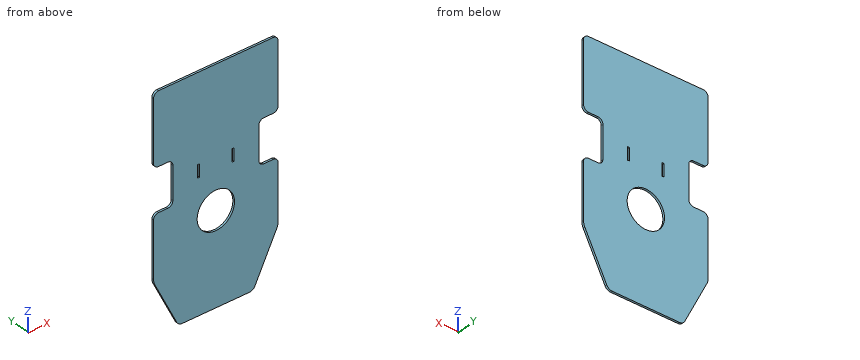
from build123d import *

# Parameters (mm, degrees)
RESSALTO_EXTRUS_O1_DEPTH = 0.8
FILETE6_R                = 2
CHANFRO3_SIZE            = 10
CHANFRO3_SIZE2           = 20
CHANFRO4_SIZE            = 20
CHANFRO4_SIZE2           = 10
FILETE7_R                = 2.5
ESBO_O7_R                = 7.5
CORTE_EXTRUS_O1_DEPTH    = 0.8
CAVIDADE1_START          = -7.3
CAVIDADE1_OUTLINE_W      = 0.8
CAVIDADE1_OUTLINE_H      = 5
CAVIDADE1_DEPTH          = 0.8
CAVIDADE1_START_2        = 6.5
CAVIDADE1_2_OUTLINE_W    = 0.8
CAVIDADE1_2_OUTLINE_H    = 5
CAVIDADE1_2_DEPTH        = 0.8
FILETE8_R                = 5


# Read off the part's stored shape, not the designer's step: Cavidade1
with BuildPart() as part:
    # Esboço1 → Ressalto-extrusão1 (new body)
    with BuildSketch(Plane(origin=(0, 0, 0), x_dir=(1, 0, 0), z_dir=(0, 1, 0))):
        Polygon((-17.25, 45), (-25, 45), (-25, 90), (0, 90), (0, 0), (-25, 0), (-25, 28), (-17.25, 28), align=None)
    ressalto_extrus_o1 = extrude(amount=RESSALTO_EXTRUS_O1_DEPTH)

    # Espelhar8: Ressalto-extrusão1 across plane
    add(ressalto_extrus_o1.mirror(Plane(origin=(0, 0, 0), x_dir=(0, 0, 1), z_dir=(1, 0, 0))))

    # Filete6
    filete6_edges = [part.edges().sort_by_distance(p)[0] for p in [
        (-25, 0.4, -45),
        (-17.25, 0.4, -45),
        (-17.25, 0.4, -28),
        (-25, 0.4, -28),
        (-25, 0.4, 0),
        (25, 0.4, 0),
        (25, 0.4, -28),
        (17.25, 0.4, -28),
        (17.25, 0.4, -45),
        (25, 0.4, -45),
    ]]
    fillet(filete6_edges, radius=FILETE6_R)

    # Chanfro3
    chanfro3_edges = [part.edges().sort_by_distance(p)[0] for p in [
        (-25, 0.4, -90),
    ]]
    chanfro3_side = [part.faces().sort_by_distance(p)[0] for p in [
        (0, 0.4, -90),
    ]]
    chamfer(chanfro3_edges, length=CHANFRO3_SIZE, length2=CHANFRO3_SIZE2, reference=chanfro3_side[0])

    # Chanfro4
    chanfro4_edges = [part.edges().sort_by_distance(p)[0] for p in [
        (25, 0.4, -90),
    ]]
    chanfro4_side = [part.faces().sort_by_distance(p)[0] for p in [
        (25, 0.4, -68.5),
    ]]
    chamfer(chanfro4_edges, length=CHANFRO4_SIZE, length2=CHANFRO4_SIZE2, reference=chanfro4_side[0])

    # Filete7
    filete7_edges = [part.edges().sort_by_distance(p)[0] for p in [
        (-15, 0.4, -90),
        (15, 0.4, -90),
    ]]
    fillet(filete7_edges, radius=FILETE7_R)

    # Esboço7 → Corte-extrusão1 (cut)
    with BuildSketch(Plane(origin=(0, 0.8, 0), x_dir=(1, 0, 0), z_dir=(0, 1, 0))):
        with Locations(Location((0, 54, 0), (0, 0, 270))):
            Circle(ESBO_O7_R)
    extrude(amount=-CORTE_EXTRUS_O1_DEPTH, mode=Mode.SUBTRACT)

    # Cavidade1 outline → Cavidade1 (cut)
    with BuildSketch(Plane.YZ.offset(CAVIDADE1_START)):
        with Locations((0.4, -36.5)):
            Rectangle(CAVIDADE1_OUTLINE_W, CAVIDADE1_OUTLINE_H)
    extrude(amount=CAVIDADE1_DEPTH, mode=Mode.SUBTRACT)

    # Cavidade1 2 outline → Cavidade1 2 (cut)
    with BuildSketch(Plane.YZ.offset(CAVIDADE1_START_2)):
        with Locations((0.4, -36.5)):
            Rectangle(CAVIDADE1_2_OUTLINE_W, CAVIDADE1_2_OUTLINE_H)
    extrude(amount=CAVIDADE1_2_DEPTH, mode=Mode.SUBTRACT)

    # Filete8
    filete8_edges = [part.edges().sort_by_distance(p)[0] for p in [
        (-25, 0.4, -70),
        (25, 0.4, -70),
    ]]
    fillet(filete8_edges, radius=FILETE8_R)


solid = part.part
Could you check a few things on this model? Use its own coordinates, in mm. Give positions to 0.01 mm unless a question says otherwise; leave off trailing zeros. Order: outer loops, then holes, each group sorted by start corner. A loop starts at its lowest first (then second) coordinate and runs counter-clockwise, first axis right, second up.
Item 1: If we section it at B-B, the plane z = -54: Write out the boundary of the cut face in (x, y), plus the area to 3 significant figures.
Item 2: If we section it at D-D, the plane z = -32: Write out the boundary of the cut face in (x, y), plus the area to 3 significant figures.
Item 3: If we section it at A-A, the plane x = 0: Write out the boundary of the cut face in (y, z), plus the area to 3 significant figures.
Item 4: I need wall thicknesses on line 1 (X direction, y = 0.35, z = -54); line 2 (Z direction, x = -20.5, y = 0.4); line 3 (X direction, y = 0.15, z = -55.5). Which ranges of each line are inside material? Lowest first, please.
Item 5: If we section it at C-C, the plane y = 0.2: Count the separate pieces of the cut face and the enclosed holes in it, plus the area to 3 significant figures.
Values:
1. outline: (-25, 0) - (-7.5, 0) - (-7.5, 0.8) - (-25, 0.8) - close; (7.5, 0) - (25, 0) - (25, 0.8) - (7.5, 0.8) - close
1. area: 28.0 mm2
2. outline: (-17.25, 0) - (17.25, 0) - (17.25, 0.8) - (-17.25, 0.8) - close
2. area: 27.6 mm2
3. outline: (0, -90) - (0.8, -90) - (0.8, -61.5) - (0, -61.5) - close; (0, -46.5) - (0.8, -46.5) - (0.8, 0) - (0, 0) - close
3. area: 60.0 mm2
4. line 1: x = -25 to -7.5, 7.5 to 25
4. line 2: z = -79 to -45, -28 to 0
4. line 3: x = -25 to -7.35, 7.35 to 25
5. separate pieces: 1
5. enclosed holes: 3
5. area: 3,850 mm2
